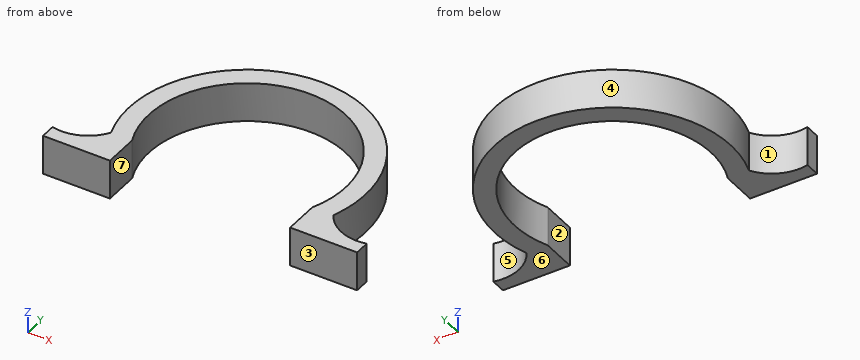
```python
from build123d import *

# Parameters (mm, degrees)
BOSS_EXTRUDE2_DEPTH = 12.7
BOSS_EXTRUDE3_DEPTH = 12.7


with BuildPart() as part:
    # Sketch3 → Boss-Extrude2 (new body)
    with BuildSketch(Plane.XY):
        with BuildLine():
            Line((-35.921024484, -12.7), (-29.099355663, -12.7))
            ThreePointArc((-29.099355663, -12.7), (0, 31.75), (29.099355663, -12.7))
            Line((29.099355663, -12.7), (35.921024484, -12.7))
            ThreePointArc((35.921024484, -12.7), (0, 38.1), (-35.921024484, -12.7))
        make_face()
    extrude(amount=BOSS_EXTRUDE2_DEPTH)

    # Sketch4 → Boss-Extrude3 (add)
    with BuildSketch(Plane(origin=(0, 0, 0), x_dir=(-1, 0, 0), z_dir=(0, 0, -1))):
        with BuildLine():
            Line((-29.099355663, -12.7), (-29.099355663, -23.876))
            Line((-29.099355663, -23.876), (-50.714755663, -23.876))
            Line((-50.714755663, -23.876), (-50.714755663, -19.05))
            ThreePointArc((-50.714755663, -19.05), (-42.288257842, -18.27375629), (-35.921024484, -12.7))
            Line((-35.921024484, -12.7), (-29.099355663, -12.7))
        make_face()
        with BuildLine():
            Line((29.099355663, -12.7), (29.099355663, -23.876))
            Line((29.099355663, -23.876), (50.714755663, -23.876))
            Line((50.714755663, -23.876), (50.714755663, -19.05))
            ThreePointArc((50.714755663, -19.05), (42.288257842, -18.27375629), (35.921024484, -12.7))
            Line((35.921024484, -12.7), (29.099355663, -12.7))
        make_face()
    extrude(amount=-BOSS_EXTRUDE3_DEPTH)


solid = part.part
```
Geometry check sheet. Reference: the model listing, model coordinates, mm. Face numbers are marked on the shaded views. A direction names the side the tool comes from. Round coordinates to 2 decimals unless told otherwise and drop trailing zeros. Loops run counter-clockwise (first coordinate to the right, second up) from the corner with the lowest first, then second, coordinate; pieces in that order, holes last. Notation, with made-up numbers: (4, -23.5) - (36, -23.5) arc R24 cw to (36, -11.5) - close; hole circle Ø8 at (43, 39.5). An arc over 180 degrees is marked (long way). Write each question's results on one line, items separated by ' | '. Start each with the question number.
Q1. Gauge pin test, flat ends, axial feed: P1, Ø1, axis at y = -7, z = 7.5, coming from the -X side; P2, Ø1, axis at y = 29.5, z = 2, coming from the -X side; P3, Ø5, axis at y = 16, z = 10, coming from the +X side. Record the tip position at first contact, or that the pin passes through.
Q2. Cross-section at B-B on z = 5.5. Enter the section's corners in (x, y).
Q3. Release check for a two-part mould opening along X. For the marked faces 1, 2, 3 and 4 record: +X half, -X half, draft (parallel to the pull), parting line (faces both ways), or undercut.
Q4. Cross-section at D-D on y = 15. Enter the section's corners in (x, z).
Q5. Cross-section at C-C on x = 0. Enter the section's corners in (y, z), and give its area (3 significant figures).
Q6. Thickness scan on line 1 (X direction, y = 0, z = 5); line 2 (X direction, y = 23, z = 10.5); line 3 (Y direction, x = -33.5, z = 8). Record the ranges inside material, lowest first. Write a range as [from, to].
Q7. Access from +Z, -Z, +X, -X, +Y, -Y to the whole of each face (thin tool, end or side, straight path). Record for the marked faces 5, 6 and 7.
Q8. Cross-section at A-A on y = 0. Enter the section's corners in (x, z), and give its area (3 significant figures).
Answers below:
1) P1: stops at x = -37.54 | P2: stops at x = -24.71 | P3: stops at x = 35.63
2) outline: (-50.71, -23.88) - (-29.1, -23.88) - (-29.1, -12.7) arc R31.75 cw (long way) to (29.1, -12.7) - (29.1, -23.88) - (50.71, -23.88) - (50.71, -19.05) arc R13.72 cw to (35.92, -12.7) arc R38.1 ccw (long way) to (-35.92, -12.7) arc R13.72 cw to (-50.71, -19.05) - close
3) face 1: undercut | face 2: undercut | face 3: draft | face 4: parting line
4) outline: (-35.02, 0) - (-27.98, 0) - (-27.98, 12.7) - (-35.02, 12.7) - close; (27.98, 0) - (35.02, 0) - (35.02, 12.7) - (27.98, 12.7) - close
5) outline: (31.75, 0) - (38.1, 0) - (38.1, 12.7) - (31.75, 12.7) - close | area: 80.6 mm²
6) line 1: x = [-38.1, -31.75], [31.75, 38.1] | line 2: x = [-30.37, -21.89], [21.89, 30.37] | line 3: y = [-23.88, 18.15]
7) face 5: +Z, -Z | face 6: -Z, +X, -X, +Y, -Y | face 7: +Z, -Z, -Y
8) outline: (-38.1, 0) - (-31.75, 0) - (-31.75, 12.7) - (-38.1, 12.7) - close; (31.75, 0) - (38.1, 0) - (38.1, 12.7) - (31.75, 12.7) - close | area: 161 mm²
